```python
from build123d import *

# Parameters (mm, degrees)
BOSS_EXTRUDE1_DEPTH = 6.35


with BuildPart() as part:
    # Sketch2 → Boss-Extrude1 (new body)
    with BuildSketch(Plane.XY):
        with BuildLine():
            Line((-0.14988496, 38.540888918), (6.080919163, 36.469296285))
            Line((6.080919163, 36.469296285), (8.602283556, 38.398893807))
            Line((8.602283556, 38.398893807), (13.346918999, 36.821416544))
            Line((13.346918999, 36.821416544), (10.825554606, 34.891819022))
            Line((10.825554606, 34.891819022), (17.056358729, 32.820226388))
            Line((17.056358729, 32.820226388), (-62.447694199, -12.10770477))
            Line((-62.447694199, -12.10770477), (-62.447694199, -4.16341339))
            Line((-62.447694199, -4.16341339), (-65.622694199, -4.16341339))
            Line((-65.622694199, -4.16341339), (-65.622694199, -7.33841339))
            Line((-65.622694199, -7.33841339), (-69.654994999, -7.33841339))
            Line((-69.654994999, -7.33841339), (-69.654994999, -4.16341339))
            ThreePointArc((-69.654994999, -4.16341339), (-68.473961439, -1.312146151), (-65.622694199, -0.13111259))
            Line((-65.622694199, -0.13111259), (-62.447694199, -0.13111259))
            Line((-62.447694199, -0.13111259), (-62.447694199, 6.780877989))
            Line((-62.447694199, 6.780877989), (-0.14988496, 38.540888918))
        make_face()
    extrude(amount=BOSS_EXTRUDE1_DEPTH)


solid = part.part
```
Geometry: final body of the model. Coordinates: model frame, mm. A direction names the side the tool comes from. Round coordinates to 2 decimals unless told otherwise and drop trailing zeros. Order: outer loops, then holes, each group sorted by start corner. A loop starts at its lowest first (then second) coordinate and runs counter-clockwise, first axis right, second up. Notation, with made-up numbers: M -25.75,53 L 18.25,53 A20 cw 18.25,63 Z; hole C 2,-21 d7. An arc over 180 degrees is marked long. One line per item, written item: value.
(1) Pin query (flat end, axial travel): P1, Ø1, axis at x = -63.5, z = 2, coming from the -Y side; P2, Ø3, axis at x = -68.5, z = 2, coming from the -Y side; P3, Ø2.5, axis at x = -63.5, z = 2, coming from the +Y side. Return the tip coordinate at first contact, or that it passes through.
Result sheet:
P1: y = -4.16
P2: y = -7.34
P3: y = 6.88
(2) Cut plane C-C (x = 7). Return the cut outline in (y, z), and give its area (3 significant figures).
Result sheet:
outline: M 27.14,0 L 37.17,0 L 37.17,6.35 L 27.14,6.35 Z
area: 63.7 mm2
(3) Line query: probe 1 along Y at (x, z) = (-65.5, 5.5); probe 2 along X at (y, z) = (-6.5, 2.5) (3 decimals); probe 3 along Y at (x, z) = (11, 5). Output: solid intervals per line, ascending. Write a range as [from, to].
Result sheet:
probe 1: [-4.16, -0.13]
probe 2: [-69.655, -65.623], [-62.448, -52.524]
probe 3: [29.4, 34.83], [35.03, 37.6]
(4) Cut plane A-A (z = 4.25). Return the cut outline in (x, y) (3 decimals).
Result sheet:
outline: M -69.655,-7.338 L -65.623,-7.338 L -65.623,-4.163 L -62.448,-4.163 L -62.448,-12.108 L 17.056,32.82 L 10.826,34.892 L 13.347,36.821 L 8.602,38.399 L 6.081,36.469 L -0.15,38.541 L -62.448,6.781 L -62.448,-0.131 L -65.623,-0.131 A4.032 ccw -69.655,-4.163 Z
(5) Cut plane B-B (y = 28). Return the cut outline in (x, z).
Result sheet:
outline: M -20.83,0 L 8.53,0 L 8.53,6.35 L -20.83,6.35 Z
(6) Reachability of faces 5 (the flat face through (-64, -0.131, 3)), 6 (the flat face through (-68, -7.338, 3)), 7 (the flat face through (13.9, 33.87, 3.13)), 8 (the flat face through (7.3, 37.4, 3.1)), 9 (the flat face through (-62.448, -8, 3)) from +Z, -Z, +X, -X, +Y, -Y: full face, straight path, thin tool, end or side. Return the list, or none.
Result sheet:
face 5: +Z, -Z, -X, +Y
face 6: +Z, -Z, -X, -Y
face 7: +Z, -Z, +X
face 8: +Z, -Z, +Y
face 9: +Z, -Z, -Y
(7) Pull-direction query (X, two-part tool) for faces 1 (the flat face through (-62.448, 3, 3)), 2 (the flat face through (-64, -4.163, 3)), 3 (the flat face through (2.92, 37.52, 3.13)), 4 (the flat face through (-29, 15, 6.35)); classes: pulls with the +X half, pulls with the -X half, needs draft (parallel to the pull), parting line crosses it, or undercut.
Result sheet:
face 1: pulls with the -X half
face 2: undercut
face 3: undercut
face 4: needs draft
